```python
from build123d import *

# Parameters (mm, degrees)
SKETCH1_W           = 800.1
SKETCH1_H           = 311.15
BOSS_EXTRUDE1_DEPTH = 1.5875
CUT_EXTRUDE1_DEPTH  = 859.477963098


with BuildPart() as part:
    # Sketch1 → Boss-Extrude1 (new, symmetric)
    with BuildSketch(Plane.XY):
        with Locations((400.05, 155.575)):
            Rectangle(SKETCH1_W, SKETCH1_H)
    extrude(amount=BOSS_EXTRUDE1_DEPTH, both=True)

    # Sketch2 → Cut-Extrude1 (cut, through all)
    with BuildSketch(Plane.XY.offset(1.5875)):
        with BuildLine():
            ThreePointArc((73.799735787, 80.288462856), (136.885533296, 116.716615986), (193.450443102, 162.621290763))
            Line((193.450443102, 162.621290763), (334.279123198, 296.679860281))
            ThreePointArc((334.279123198, 296.679860281), (350.98014935, 307.39838407), (370.46697579, 311.15))
            Line((370.46697579, 311.15), (0, 311.15))
            Line((0, 311.15), (0, 0))
            ThreePointArc((0, 0), (29.11988212, 47.295456823), (73.799735787, 80.288462856))
        make_face()
        with BuildLine():
            Line((800.1, 311.15), (370.46697579, 311.15))
            ThreePointArc((370.46697579, 311.15), (390.494645186, 306.92285828), (407.105710958, 294.962558849))
            Line((407.105710958, 294.962558849), (457.816588668, 239.285045675))
            ThreePointArc((457.816588668, 239.285045675), (467.985750385, 264.275368722), (493.30296488, 273.60096502))
            ThreePointArc((493.30296488, 273.60096502), (518.828524121, 268.832657986), (542.448186048, 258.0436591))
            Line((542.448186048, 258.0436591), (800.1, 99.941615608))
            Line((800.1, 99.941615608), (800.1, 311.15))
        make_face()
    extrude(amount=-CUT_EXTRUDE1_DEPTH, mode=Mode.SUBTRACT)


solid = part.part
```
Part model, mm, in its own coordinate system. Round coordinates to 2 decimals unless told otherwise and drop trailing zeros. Loops run counter-clockwise (first coordinate to the right, second up) from the corner with the lowest first, then second, coordinate; pieces in that order, holes last.
Item 1: Cut at A-A, the plane z = 0.6. Give the cut face in (x, y) (3 decimals).
Item 2: Drop a flat-ended pin along its axis: P1, Ø8, axis at x = 443.5, y = 263, coming from the +Z side. Give the stop position or say it passes through.
Item 3: Cut at C-C, the plane x = 396. Give the cut face in (y, z).
Item 4: Mould opens along X. For faces 1 (the face through (28.592, 46.718, 0.022)), 2 (the face through (467.708, 264.003, 0.022)), 3 (the face through (394, 123, -1.588)), 4 (the face through (432.11, 267.51, 0.02)) say: +X half, -X half, draft (parallel to the pull), parting line (faces both ways), or undercut.
Item 5: Drill centre lines: line 1 (X direction, y = 243.5, z = 0.8); line 2 (X direction, y = 258, z = -1.35); line 3 (Y direction, x = 624, z = 0.45). Where is each one in solid material? Low to high.
Item 6: Cut at B-B, the plane y = 266. Give the cut face in (x, z).
Item 7: Cut at D-D, the plane y = 193. Give the cut face in (x, z), then the cut area to 3 significant figures.
A:
1. outline: (0, 0) - (800.1, 0) - (800.1, 99.942) - (542.448, 258.044) arc R106.773 ccw to (493.303, 273.601) arc R33.405 ccw to (457.817, 239.285) - (407.106, 294.963) arc R49.558 ccw to (370.467, 311.15) arc R52.486 ccw to (334.279, 296.68) - (193.45, 162.621) arc R461.33 cw to (73.8, 80.288) arc R145.961 ccw to start
2. P1: passes through
3. outline: (0, -1.59) - (304.07, -1.59) - (304.07, 1.59) - (0, 1.59) - close
4. face 1: -X half
4. face 2: undercut
4. face 3: draft
4. face 4: undercut
5. line 1: x = 278.41 to 453.98, 457.96 to 566.15
5. line 2: x = 293.65 to 440.77, 462.9 to 542.52
5. line 3: y = 0 to 208
6. outline: (302.05, -1.59) - (433.48, -1.59) - (433.48, 1.59) - (302.05, 1.59) - close; (469.91, -1.59) - (526.69, -1.59) - (526.69, 1.59) - (469.91, 1.59) - close
7. outline: (225.36, -1.59) - (648.45, -1.59) - (648.45, 1.59) - (225.36, 1.59) - close
7. area: 1,340 mm2
